The model under review builds one solid part; all positions refer to its coordinate system, in mm. Coordinates: 2 decimals unless noted, no trailing zeros. Order: outer loops, then holes, each group sorted by start corner. A loop starts at its lowest first (then second) coordinate and runs counter-clockwise, first axis right, second up.
from build123d import *

# Parameters (mm, degrees)
SKETCH_1_R      = 2.8
EXTRUDE_1_DEPTH = 3
EXTRUDE_2_DEPTH = 1.5
SKETCH_2_R      = 1.5
EXTRUDE_3_DEPTH = 75


with BuildPart() as part:
    # Sketch 1 → Extrude 1 (new body)
    with BuildSketch(Plane(origin=(0, 0, 0), x_dir=(1, 0, 0), z_dir=(0, 1, 0))):
        with Locations(Location((0, 0, 0), (0, 0, 270))):
            Circle(SKETCH_1_R)
        Polygon((1.25, -0.721687836), (1.25, 0.721687836), (0, 1.443375673), (-1.25, 0.721687836), (-1.25, -0.721687836), (0, -1.443375673), align=None, mode=Mode.SUBTRACT)
    extrude(amount=EXTRUDE_1_DEPTH)

    # Sketch 1_2 → Extrude 2 (add)
    with BuildSketch(Plane(origin=(0, 0, 0), x_dir=(1, 0, 0), z_dir=(0, 1, 0))):
        Polygon((-1.25, -0.721687836), (0, -1.443375673), (1.25, -0.721687836), (1.25, 0.721687836), (0, 1.443375673), (-1.25, 0.721687836), align=None)
    extrude(amount=EXTRUDE_2_DEPTH)

    # Sketch 2 → Extrude 3 (add)
    with BuildSketch(Plane.XZ):
        with Locations(Location((0, 0, 0), (0, 0, 270))):
            Circle(SKETCH_2_R)
    extrude(amount=EXTRUDE_3_DEPTH)


solid = part.part
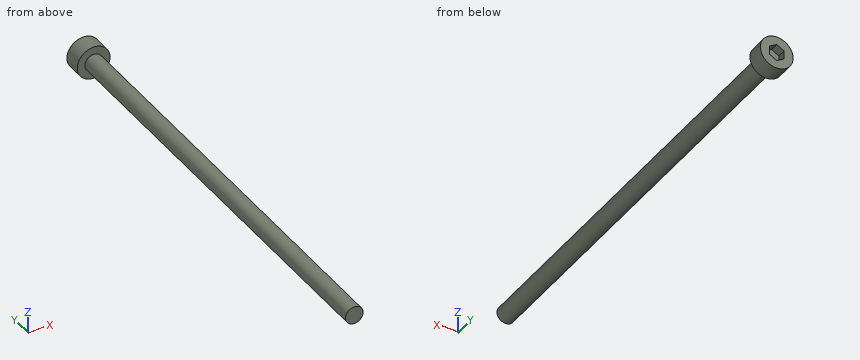
(1) Consider section A-A (z = 0). Give the boundary of the cut face in (x, y).
(2) Consider section B-B (y = -52.5). Give the boundary of the cut face in (x, z), then the cut area to 3 significant figures.
(3) Insertion check: pin 1 Ø2 at (x, y) = (1.5, -44) entering from -Z; pin 2 Ø1.5 at (y, z) = (-12.5, 1.5) entering from -X; pin 3 Ø0.8 at (x, z) = (0, -0.5) entering from +Y. Each pin has a flat end and moves straight along its axis. Give the tip position at first contact, or say it passes through.
(4) Wall thickness on line 1 (Y direction, x = 0.05, z = -2.05); line 2 (Y direction, x = -0.75, z = -0.75); line 3 (X direction, y = -65, z = -0.05): over which ranges is each line inside the solid? List them lowest first.
Findings:
1. outline: (-2.8, 0) - (-1.5, 0) - (-1.5, -75) - (1.5, -75) - (1.5, 0) - (2.8, 0) - (2.8, 3) - (1.25, 3) - (1.25, 1.5) - (-1.25, 1.5) - (-1.25, 3) - (-2.8, 3) - close
2. outline: circle Ø3 at (0, 0)
2. area: 7.07 mm2
3. pin 1: stops at z = -1.41
3. pin 2: stops at x = -1.3
3. pin 3: stops at y = 1.5
4. line 1: y = 0 to 3
4. line 2: y = -75 to 1.5
4. line 3: x = -1.5 to 1.5
